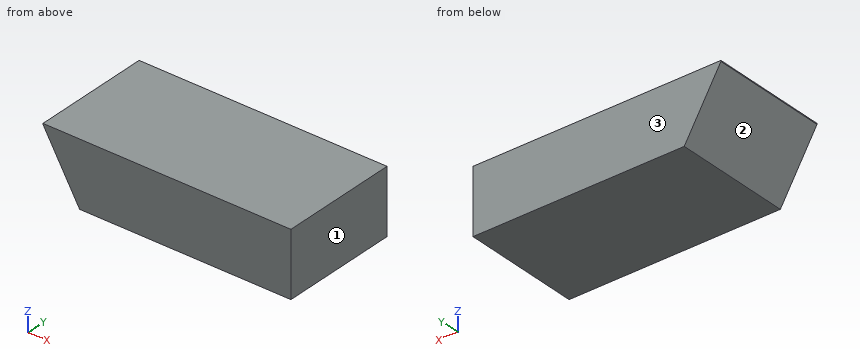
from build123d import *

# Parameters (mm, degrees)
BOX016_W               = 250
BOX016_H               = 120
BOX016_DEPTH           = 65
BOX016_PLACEMENT_ANGLE = 60
BOX017_W               = 250
BOX017_H               = 120
BOX017_DEPTH           = 65
CUT009_PLACEMENT_ANGLE = 180


with BuildPart() as box016:
    # Box016 → Box016 (new body)
    with BuildSketch(Plane.XY):
        with Locations((125, 60)):
            Rectangle(BOX016_W, BOX016_H)
    extrude(amount=BOX016_DEPTH)


with BuildPart() as box016_1:
    # Box016 placement: moved
    add(box016.part.moved(Location((187.927513, 0, 108.5))).rotate(Axis((187.927513, 0, 108.5), (0, 1, 0)), BOX016_PLACEMENT_ANGLE))


with BuildPart() as cut009:
    # Box017 → Box017 (new body)
    with BuildSketch(Plane.XY):
        with Locations((125, 60)):
            Rectangle(BOX017_W, BOX017_H)
    extrude(amount=BOX017_DEPTH)

    # Cut009: cut Box016
    add(box016_1.part, mode=Mode.SUBTRACT)


with BuildPart() as cut009_1:
    # Cut009 placement: moved
    add(cut009.part.moved(Location((469, 0, 64))).rotate(Axis((469, 0, 64), (0, 1, 0)), CUT009_PLACEMENT_ANGLE))


solid = cut009_1.part
Can you work these out from the model? Positions are in its coordinate system, mm. Face numbers are marked on the shaded views. Round coordinates to 2 decimals unless told otherwise and drop trailing zeros. Loops run counter-clockwise (first coordinate to the right, second up) from the corner with the lowest first, then second, coordinate; pieces in that order, holes last. Notation, with made-up numbers: (-39, 68) - (-6, 68) arc R22 ccw to (-6, 93) - close; hole circle Ø6 at (23.5, 83). An arc over 180 degrees is marked (long way). Use CSV: the item, a comma, the result in double quotes. Start each with the question number.
1) We'd pull the mould along X, two halves only. Please class the marked faces 1, 2 and 3: released by +X, released by -X, zero draft, split by the parting line, or undercut.
2) If we section it at B-B on z = 26: Write out the boundary of the cut face in (x, y).
3) If we section it at A-A on y = 92.5: Write out the boundary of the cut face in (x, z), plus the area to 3 significant figures.
4) Please list where these lines run through material, in increasing order: probe 1 along X at (y, z) = (89.5, 13.5); probe 2 along X at (y, z) = (34.5, 43). Write a range as [from, to].
5) If we section it at C-C on x = 239: Write out the boundary of the cut face in (y, z).
6) For pin 1 Ø1 at (x, z) = (262.5, 32) entering from -Y, with a flat end and sliding along its axis, tell me the tip position at first contact or that it passes through.
Geometry results:
1,face 1,"released by +X"
1,face 2,"released by -X"
1,face 3,"zero draft"
2,outline,"(240.37, 0) - (469, 0) - (469, 120) - (240.37, 120) - close"
3,outline,"(219, 63.01) - (255.96, -1) - (469, -1) - (469, 64) - (219, 64) - close"
3,area,"15,100 mm2"
4,probe 1,"x = [247.59, 469]"
4,probe 2,"x = [230.55, 469]"
5,outline,"(0, 28.37) - (120, 28.37) - (120, 64) - (0, 64) - close"
6,pin 1,"stops at y = 0"
